```python
from build123d import *

# Parameters (mm, degrees)
SKETCH2_W           = 53.4
SKETCH2_H           = 104.3
BOSS_EXTRUDE1_DEPTH = 9
SKETCH3_R           = 1.96
CUT_EXTRUDE1_DEPTH  = 60.274889287
SKETCH4_W           = 26.134
SKETCH4_H           = 2
BOSS_EXTRUDE2_DEPTH = 8
FILLET1_R           = 0.5
CUT_EXTRUDE3_DEPTH  = 3
SKETCH8_W           = 53.4
SKETCH8_H           = 9
BOSS_EXTRUDE4_DEPTH = 2
SKETCH9_W           = 37.2
SKETCH9_H           = 1.98
BOSS_EXTRUDE5_DEPTH = 14.4
BOSS_EXTRUDE6_DEPTH = 3
FILLET2_R           = 5
SKETCH13_W          = 53.4
SKETCH13_H          = 9
BOSS_EXTRUDE8_DEPTH = 5
FILLET3_R           = 5


with BuildPart() as part:
    # Sketch2 → Boss-Extrude1 (new body)
    with BuildSketch(Plane.XY):
        Rectangle(SKETCH2_W, SKETCH2_H)
    extrude(amount=BOSS_EXTRUDE1_DEPTH)

    # Sketch3 → Cut-Extrude1 (cut, through all)
    with BuildSketch(Plane(origin=(0, 0, 0), x_dir=(-1, 0, 0), z_dir=(0, 0, -1))):
        with Locations((24.1, 38.21)):
            Circle(SKETCH3_R)
        with Locations((-24.16, 36.91)):
            Circle(SKETCH3_R)
        with Locations((-8.92, -13.89)):
            Circle(SKETCH3_R)
        with Locations((19.02, -13.89)):
            Circle(SKETCH3_R)
    extrude(amount=-CUT_EXTRUDE1_DEPTH, mode=Mode.SUBTRACT)

    # Sketch4 → Boss-Extrude2 (add)
    with BuildSketch(Plane.XY.offset(9)):
        with Locations((-7.427, -5.35)):
            Rectangle(SKETCH4_W, SKETCH4_H)
    extrude(amount=BOSS_EXTRUDE2_DEPTH)

    # Fillet1
    fillet1_edges = [part.edges().sort_by_distance(p)[0] for p in [
        (-7.427, -6.35, 9),
    ]]
    fillet(fillet1_edges, radius=FILLET1_R)

    # Sketch6 → Cut-Extrude3 (cut)
    with BuildSketch(Plane.XY.offset(9)):
        Polygon((-21.3, 36.593419246), (-21.3, 39.826580754), (-24.1, 41.443161507), (-26.9, 39.826580754), (-26.9, 36.593419246), (-24.1, 34.976838493), align=None)
        Polygon((26.96, 35.293419246), (26.96, 38.526580754), (24.16, 40.143161507), (21.36, 38.526580754), (21.36, 35.293419246), (24.16, 33.676838493), align=None)
        Polygon((-16.22, -15.506580754), (-16.22, -12.273419246), (-19.02, -10.656838493), (-21.82, -12.273419246), (-21.82, -15.506580754), (-19.02, -17.123161507), align=None)
        Polygon((11.72, -15.506580754), (11.72, -12.273419246), (8.92, -10.656838493), (6.12, -12.273419246), (6.12, -15.506580754), (8.92, -17.123161507), align=None)
    extrude(amount=-CUT_EXTRUDE3_DEPTH, mode=Mode.SUBTRACT)

    # Sketch8 → Boss-Extrude4 (add)
    with BuildSketch(Plane.XZ.offset(52.15)):
        with Locations((0, 4.5)):
            Rectangle(SKETCH8_W, SKETCH8_H)
    extrude(amount=BOSS_EXTRUDE4_DEPTH)

    # Sketch9 → Boss-Extrude5 (add)
    with BuildSketch(Plane.XY.offset(9)):
        with Locations((-0.9, -53.16)):
            Rectangle(SKETCH9_W, SKETCH9_H)
    extrude(amount=BOSS_EXTRUDE5_DEPTH)

    # Sketch10 → Boss-Extrude6 (add)
    with BuildSketch(Plane.XZ.offset(54.15)):
        with BuildLine():
            Line((14.7, 20.4), (-19.5, 20.4))
            Line((-19.5, 20.4), (-19.5, 23.4))
            Line((-19.5, 23.4), (17.7, 23.4))
            ThreePointArc((17.7, 23.4), (16.821320344, 21.278679656), (14.7, 20.4))
        make_face()
    extrude(amount=-BOSS_EXTRUDE6_DEPTH)

    # Fillet2
    fillet2_edges = [part.edges().sort_by_distance(p)[0] for p in [
        (-7.427, -4.35, 9),
    ]]
    fillet(fillet2_edges, radius=FILLET2_R)

    # Sketch13 → Boss-Extrude8 (add)
    with BuildSketch(Plane.XZ.offset(54.15)):
        with Locations((0, 4.5)):
            Rectangle(SKETCH13_W, SKETCH13_H)
    extrude(amount=BOSS_EXTRUDE8_DEPTH)

    # Fillet3
    fillet3_edges = [part.edges().sort_by_distance(p)[0] for p in [
        (-0.9, -54.15, 9),
    ]]
    fillet(fillet3_edges, radius=FILLET3_R - 0.0001)  # a hair under: the kernel refuses the full size


solid = part.part
```
For this review, take the finished solid that the model builds, in its own axes (mm). A direction names the side the tool comes from. Give positions to 0.01 mm unless a question says otherwise; leave off trailing zeros. Loops run counter-clockwise (first coordinate to the right, second up) from the corner with the lowest first, then second, coordinate; pieces in that order, holes last. Notation, with made-up numbers: M -28,-35 L 8,-35 A11 ccw 8,-28 Z; hole C -23.75,-39 d9. An arc over 180 degrees is marked long. One line per item, written item: value. Start each with the question number.
Q1. Draft analysis for pull direction Y (two halves, no side actions). For faces 6 (the face through (26.7, -3, 4)), 7 (the face through (-22, 38, 6)), 8 (the face through (0, 52.15, 4)), 9 (the face through (25.45, 39.4, 7.52)), state which applies: released by +Y, released by -Y, zero draft, split by the parting line, or undercut.
Q2. For L1, parallel to Y at x = 24.16, z = 4.05; L2, parallel to Y at x = -24.1, z = 4.65; L3, parallel to Z at x = 8, y = 7.5, list the stretches that pass through material, from the lowest coordinate up.
Q3. Add section B-B (z = 11.25). Give the boundary of the cut face in (x, y), and give its area (3 significant figures).
Q4. Add section C-C (y = 22.5). Give the boundary of the cut face in (x, z), and give its area (3 significant figures).
Q5. Clearance check with flat-ended pins moving along their axes: pin 1 Ø1.5 at (y, z) = (36.5, 7) entering from +X; pin 2 Ø4.5 at (x, z) = (3, 19.5) entering from -Y; pin 3 Ø6 at (y, z) = (-1.5, 12.5) entering from -X. State where each tip first meets the part, or that it passes through.
Q6. Machinability: for faces 1 (the face through (-1, -54.15, 19)), 2 (the face through (-20.494, -5, 12)), 3 (the face through (25.41, 34.4, 7.52)), 4 (the face through (-21.3, 38, 8)), 5 (the face through (-1, -51.15, 22)), which of the approach directions +Z, -Z, +X, -X, +Y, -Y give a long, thin tool a straight path to every point of the face, cutting with its end or side? Answer none if there is none.
Reply:
1. face 6: zero draft
1. face 7: undercut
1. face 8: released by +Y
1. face 9: undercut
2. L1: -59.15 to 34.95, 38.87 to 52.15
2. L2: -59.15 to 36.25, 40.17 to 52.15
2. L3: 0 to 9
3. outline: M -20.49,-6.35 L 5.64,-6.35 L 5.64,-3.53 L -20.49,-3.53 Z; M -19.5,-54.97 L 17.7,-54.97 L 17.7,-52.17 L -19.5,-52.17 Z
3. area: 178 mm²
4. outline: M -26.7,0 L 26.7,0 L 26.7,9 L -26.7,9 Z
4. area: 481 mm²
5. pin 1: x = 21.36
5. pin 2: y = -54.15
5. pin 3: x = -20.49
6. face 1: +Z, +X, -X, -Y
6. face 2: +Z, -X, +Y, -Y
6. face 3: +Z
6. face 4: +Z, -X
6. face 5: +Z, +X, -X, +Y
